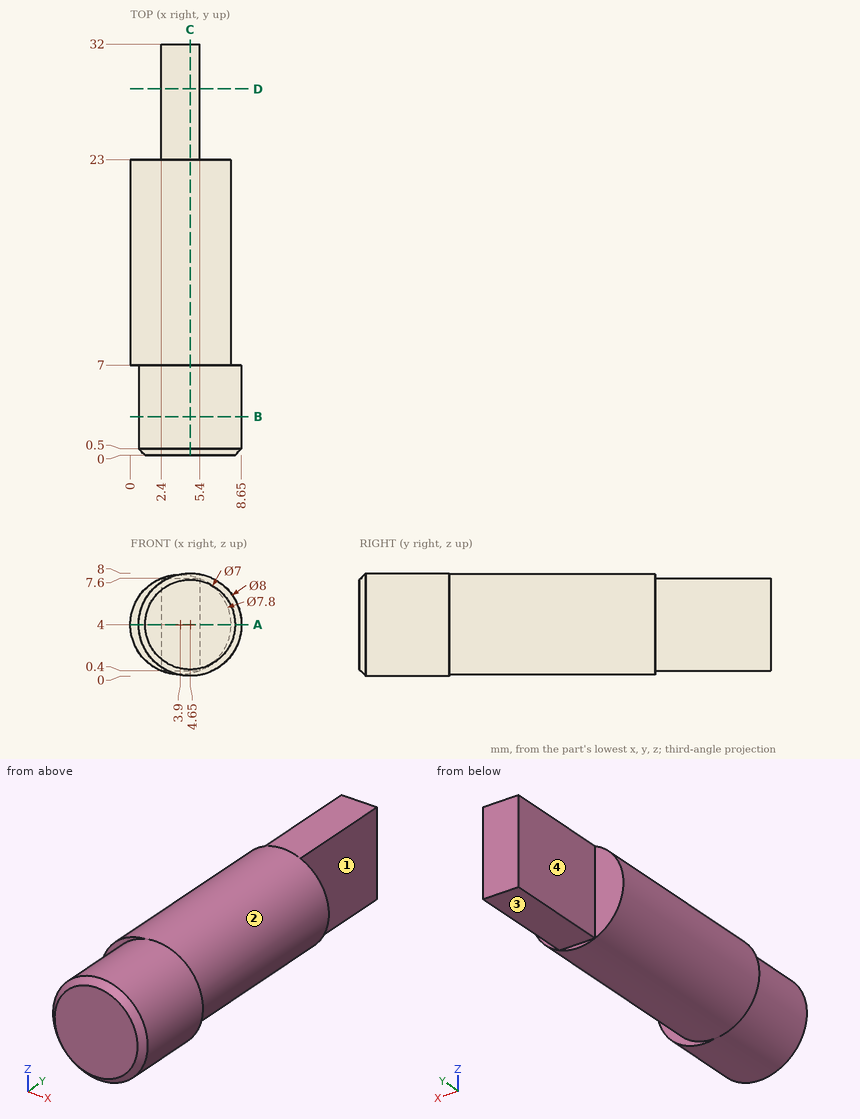
The figure shows three views and two pictorial views of one solid part (mm, origin at its lowest corner). Answer the questions. A direction names the side the tool comes from. Round coordinates to 2 decimals unless told otherwise and drop trailing zeros. Order: outer loops, then holes, each group sorted by start corner. A loop starts at its lowest first (then second) coordinate and runs counter-clockwise, first axis right, second up. Notation, with made-up numbers: (12.5, 53.25) -> (19.5, 53.25) arc R18 ccw to (19.5, 60.25) -> close; hole circle Ø9 at (88.25, 57.25). An arc over 180 degrees is marked (long way). One line per item, written item: value.
Item 1: Find section D-D, the plane y = 28.5. Give the vertices of the cut face in (x, z).
Taken from the geometry:
outline: (2.4, 0.4) -> (5.4, 0.4) -> (5.4, 7.6) -> (2.4, 7.6) -> close
Item 2: Find section C-C, the plane x = 4.65. Give the vertices of the cut face in (y, z).
Taken from the geometry:
outline: (0, 0.5) -> (0.5, 0) -> (7, 0) -> (7, 0.17) -> (23, 0.17) -> (23, 0.4) -> (32, 0.4) -> (32, 7.6) -> (23, 7.6) -> (23, 7.83) -> (7, 7.83) -> (7, 8) -> (0.5, 8) -> (0, 7.5) -> close
Item 3: For the marked faces 1, 2, 3 and 4, determine the directions among +Z, -Z, +X, -X, +Y, -Y from which every point of the face is accessible in a straight line to the end or side of a thin tool.
Taken from the geometry:
face 1: +Z, -Z, +X, +Y
face 2: +Y
face 3: -Z, +X, -X, +Y
face 4: +Z, -Z, -X, +Y
Item 4: Find section A-A, the plane z = 4. Give the vertices of the cut face in (x, y), then the cut area to 3 significant figures.
Taken from the geometry:
outline: (0, 7) -> (0.65, 7) -> (0.65, 0.5) -> (1.15, 0) -> (8.15, 0) -> (8.65, 0.5) -> (8.65, 7) -> (7.8, 7) -> (7.8, 23) -> (5.4, 23) -> (5.4, 32) -> (2.4, 32) -> (2.4, 23) -> (0, 23) -> close
area: 208 mm2
Item 5: Given P1, Ø4, axis at x = 6.5, y = 12.5, coming from the +Z side; P2, Ø1.5, axis at x = 4.5, y = 26.5, coming from the -Z side; P3, Ø1.5, axis at y = 24, z = 1.5, coming from the +X side, each flat-ended and moving along its own axis, determine where each tip first touches the part or whether it passes through.
Taken from the geometry:
P1: stops at z = 7.85
P2: stops at z = 0.4
P3: stops at x = 5.4
Item 6: Straight lines are drawn through the part: L1, parallel to Z at x = 4, y = 13; L2, parallel to Y at x = 6.75, z = 6; L3, parallel to X at y = 31, z = 6.75. For each, find the intervals that lie inside material, in ascending order.
Taken from the geometry:
L1: z = 0.1 to 7.9
L2: y = 0 to 23
L3: x = 2.4 to 5.4
Item 7: Find section B-B, the plane y = 3. Give the vertices of the cut face in (x, z).
Taken from the geometry:
outline: circle Ø8 at (4.65, 4)
